Answer from the drawing. Dimensions are ordinates in mm from the lowest x, y and z of the part. Round coordinates to 2 decimals unless told otherwise and drop trailing zeros. Order: outer loops, then holes, each group sorted by start corner. A loop starts at its lowest first (then second) coordinate and runs counter-clockwise, first axis right, second up. Notation, with made-up numbers: M 86,42.25 L 127,42.25 A10 ccw 127,53.25 Z; hole C 49,64 d3. An arc over 180 degrees is marked long. Write item = value, one per line. Start each with the question number.
(1) Straight lines are drawn through the part: probe 1 along Y at (x, z) = (2, 4.5); probe 2 along Z at (x, y) = (2.65, 47.5). For each, find the intervals that lie inside material, in ascending order. Write a range as from..to.
(2) Each of these flat-tipped pins is pushed along its axis until it touches: pin 1 (1 mm diameter, centred on x = 2, y = 54, fed in from -Z); pin 2 (2.5 mm diameter, centred on x = 1.5, z = 2, fed in from -Y); pin 3 (2.5 mm diameter, centred on x = 2.5, z = 2.5, fed in from +Y). Where does it stop, or does it pass through?
(3) A cutting plane is placed at B-B, the plane y = 12. Determine the outline of the cut face in (x, z).
(4) A cutting plane is placed at A-A, the plane x = 1.55. Determine the outline of the cut face in (y, z), and give its area (4 significant figures).
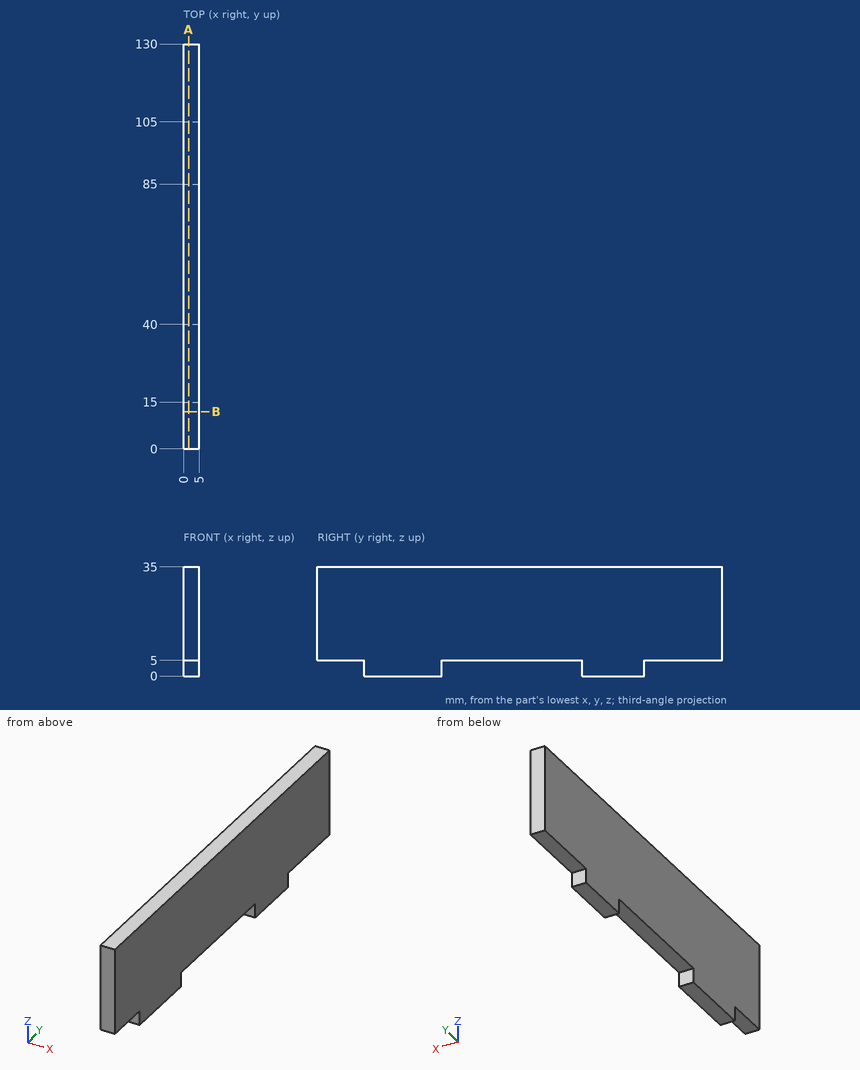
Reported:
q1.probe_1 = 15..40, 85..105
q1.probe_2 = 5..35
q2.pin_1 = 5
q2.pin_2 = 15
q2.pin_3 = 105
q3.outline = M 0,5 L 5,5 L 5,35 L 0,35 Z
q4.outline = M 0,5 L 15,5 L 15,0 L 40,0 L 40,5 L 85,5 L 85,0 L 105,0 L 105,5 L 130,5 L 130,35 L 0,35 Z
q4.area = 4,125 mm²
